Could you check a few things on this model? Use its own coordinates, in mm. Face numbers are marked on the shaded views. A direction names the side the tool comes from. Coordinates: 2 decimals unless noted, no trailing zeros. Write each loop counter-clockwise with the first axis right and the second up, starting at its lowest first coordinate (ties: lowest second). Pieces come first, ordered by that corner, then holes.
```python
from build123d import *

# Parameters (mm, degrees)
F0_R     = 33.655
F1_DEPTH = 4.826
F2_R     = 27.051
F3_DEPTH = 7.62
F4_R     = 19.05
F5_DEPTH = 12.447


with BuildPart() as f1:
    # F0 (on Top) → F1 (new body)
    with BuildSketch(Plane.XY):
        Circle(F0_R)
    extrude(amount=-F1_DEPTH)

    # F2 (on Top) → F3 (join)
    with BuildSketch(Plane.XY):
        Circle(F2_R)
    extrude(amount=F3_DEPTH)

    # F4 (on face) → F5 (cut, through all)
    with BuildSketch(Plane.XY.offset(7.62)):
        Circle(F4_R)
    extrude(amount=-F5_DEPTH, mode=Mode.SUBTRACT)


solid = f1.part
```
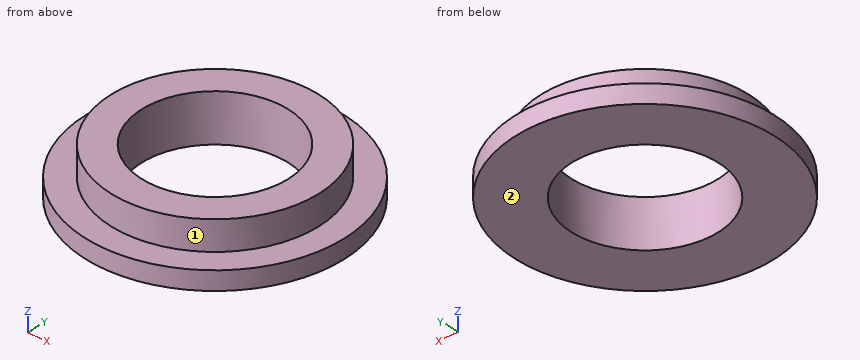
1. I want a section at D-D on x = 22.5. Please give me the cut outline in (y, z), plus the area to 3 significant figures.
Verdict:
outline: (-25.03, -4.83) - (25.03, -4.83) - (25.03, 0) - (15.02, 0) - (15.02, 7.62) - (-15.02, 7.62) - (-15.02, 0) - (-25.03, 0) - close
area: 470 mm2
2. For pin 1 (2 mm diameter, centred on x = 19.5, z = -3, fed in from +Y); pin 2 (6 mm diameter, centred on x = 4, z = -3.5, fed in from +Y); pin 3 (6 mm diameter, centred on y = 14, z = 1, fed in from +X), each with a flat end and sliding along its axis, tell me the tip position at first contact or that it passes through.
Verdict:
pin 1: stops at y = 28.11
pin 2: stops at y = 33.64
pin 3: stops at x = 31.75
3. On a 3-axis mill with a long thin cutter (end or side, diameter ignored), from which of +Z, -Z, +X, -X, +Y, -Y can I reach the whole of each face in a straight line? I mean the marked faces 1 and 2. Say none if no direction works.
Verdict:
face 1: +Z
face 2: -Z, +X, -X, +Y, -Y
4. I want a section at C-C on z = -3.25. Please give me the cut outline in (x, y) (3 decimals), plus the area to 3 significant figures.
Verdict:
outline: circle Ø67.31 at (0, 0); hole circle Ø38.1 at (0, 0)
area: 2,420 mm2
5. Please list where these lines run through material, in increasing order: line 1 along Y through (x, z) = (0, -4) (3 decimals); line 2 along Z through (x, y) = (-12, -27); line 3 along Y through (x, z) = (-0.5, 3.75).
Verdict:
line 1: y = -33.655 to -19.05, 19.05 to 33.655
line 2: z = -4.83 to 0
line 3: y = -27.05 to -19.04, 19.04 to 27.05
6. I want a section at A-A on x = 0. Please give me the cut outline in (y, z) (3 decimals).
Verdict:
outline: (-33.655, -4.826) - (-19.05, -4.826) - (-19.05, 7.62) - (-27.051, 7.62) - (-27.051, 0) - (-33.655, 0) - close; (19.05, -4.826) - (33.655, -4.826) - (33.655, 0) - (27.051, 0) - (27.051, 7.62) - (19.05, 7.62) - close
